Build history of the part. All positions in model axes, mm. Give positions to 0.01 mm unless a question says otherwise; leave off trailing zeros. Write each loop counter-clockwise with the first axis right and the second up, starting at its lowest first coordinate (ties: lowest second). Pieces come first, ordered by that corner, then holes. Notation, with made-up numbers: M -29,30.25 L 24,30.25 A18 cw 24,49.25 Z; hole C -12.5,-35.5 d2. An arc over 180 degrees is marked long. Return JSON: item names as keys, results as strings. Group by question number.
Q1. Band-saw the part on C-C, the plane y = 1.6. Give the cut face in (x, z).
Q2. Flat gauge pins, fed straight in: pin 1 Ø2.5 at (y, z) = (3, 6) entering from -X; pin 2 Ø1.5 at (y, z) = (4.5, 15.5) entering from -X; pin 3 Ø6.5 at (x, z) = (0, 0) entering from +Y; pin 4 Ø3 at (x, y) = (-28.5, 4.5) entering from -Z. Where does each tip first touch, or does it go through?
Q3. Band-saw the part on D-D, the plane x = 0. Give the cut face in (y, z), then the cut area to 3 significant figures.
Q4. Band-saw the part on B-B, the plane x = -51. Give the cut face in (y, z).
Q5. Wall check: probe 1 along X at (y, z) = (1.15, 95); probe 2 along Z at (x, y) = (-45, 1.75); probe 3 along Z at (x, y) = (0, 1.8). Give the ranges that are in metal, low to high.
Q6. Band-saw the part on A-A, the plane z = 95. Give the cut face in (x, y).
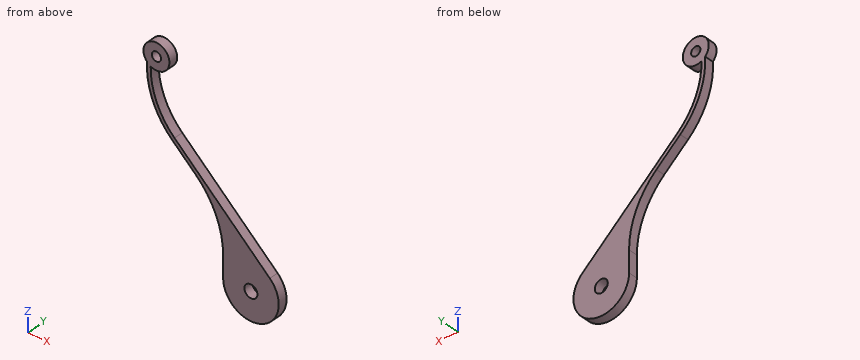
from build123d import *

# Parameters (mm, degrees)
ESQUISSE1_R      = 3.5
ESQUISSE1_R_2    = 2.5
EXTRUSION1_DEPTH = 5


with BuildPart() as part:
    # Esquisse1 → Extrusion1 (new body)
    with BuildSketch(Plane(origin=(0, 0, 0), x_dir=(1, 0, 0), z_dir=(0, 1, 0))):
        with BuildLine():
            Line((10.180478804, -11.016253961), (-41.228706345, -58.525155046))
            ThreePointArc((-41.228706345, -58.525155046), (-50.88895895, -72.244351595), (-54.072422177, -88.71864661))
            ThreePointArc((-54.072422177, -88.71864661), (-46.857537983, -100.655144285), (-56.021074344, -90.140196256))
            ThreePointArc((-56.021074344, -90.140196256), (-52.994554425, -72.099401237), (-42.586103519, -57.056321184))
            Line((-42.586103519, -57.056321184), (-29.72073238, -45.167013017))
            ThreePointArc((-29.72073238, -45.167013017), (-18.841206309, -29.882608736), (-15, -11.518997003))
            Line((-15, -11.518997003), (-15, 0))
            ThreePointArc((-15, 0), (6.012188368, 13.74240121), (10.180478804, -11.016253961))
        make_face()
        Circle(ESQUISSE1_R, mode=Mode.SUBTRACT)
        with Locations((-50.982988639, -95)):
            Circle(ESQUISSE1_R_2, mode=Mode.SUBTRACT)
    extrude(amount=EXTRUSION1_DEPTH)


solid = part.part
From the geometry:
{
 "1": {"outline": "M -56.02,90.14 A42 ccw -42.59,57.06 L -29.72,45.17 A45.82 cw -15,11.52 L -15,0 A15 ccw long 10.18,11.02 L -41.23,58.53 A40 cw -54.07,88.72 A7 ccw long Z; hole C -50.98,95 d5; hole C 0,0 d7"},
 "2": {"pin 1": "stops at x = -15", "pin 2": "stops at x = -15.24", "pin 3": "passes through", "pin 4": "stops at z = 42.43"},
 "3": {"outline": "M 0,-15 L 5,-15 L 5,-3.5 L 0,-3.5 Z; M 0,3.5 L 5,3.5 L 5,20.42 L 0,20.42 Z", "area": "142 mm^2"},
 "4": {"outline": "M 0,67.88 L 5,67.88 L 5,72.51 L 0,72.51 Z; M 0,88 L 5,88 L 5,92.5 L 0,92.5 Z; M 0,97.5 L 5,97.5 L 5,102 L 0,102 Z"},
 "5": {"probe 1": "x = -57.98 to -53.48, -48.48 to -43.98", "probe 2": "z = 59.48 to 62.52, 91.37 to 98.63", "probe 3": "z = -15 to -3.5, 3.5 to 20.42"},
 "6": {"outline": "M -57.98,0 L -53.48,0 L -53.48,5 L -57.98,5 Z; M -48.48,0 L -43.98,0 L -43.98,5 L -48.48,5 Z"}
}
